Geometry: final body of the model. Coordinates: model frame, mm. A direction names the side the tool comes from. Coordinates: 2 decimals unless noted, no trailing zeros. Order: outer loops, then holes, each group sorted by start corner. A loop starts at its lowest first (then second) coordinate and runs counter-clockwise, first axis right, second up. Notation, with made-up numbers: M -25.5,57 L 2.5,57 A10 cw 2.5,76 Z; hole C -13.75,-12.5 d8. An arc over 180 degrees is marked long. Use CSV: the item, a comma, the result in double quotes. Start each with the question number.
1. Pull-direction query (Y, two-part tool) for faces 3 (the flat face through (0, 64, -6)), 4 (the flat face through (4.2, 0, 0.2)), 5 (the cylindrical face through (8.99, 7.24, 0.49)); classes: pulls with the +Y half, pulls with the -Y half, needs draft (parallel to the pull), parting line crosses it, or undercut.
2. Set-up query: faces 1 (the flat face through (1, 64, -7)), 2 (the flat face through (7, 64, 1)). Return all of +Z, -Z, +X, -X, +Y, -Y with unobstructed straight access to the full face (end or side cutting, diameter ignored); none if empty.
3. Material intervals for line 1 (Y direction, x = 8, z = 0.85); line 2 (Z direction, x = 3.5, y = 77.5), sorted ascending.
4. First-contact query: P1, Ø7, axis at y = 94.5, z = -4.5, coming from the +X side; P2, Ø4, axis at x = 5.5, y = 92.5, coming from the -Z side. Flat tips, straight axial feed; report the tip coordinate or a pass-through.
5. Section query B-B on y = 8. Return the cut outline in (x, z), and give its area (3 significant figures).
6. Section query A-A on x = 8. Return the cut outline in (y, z).
7. Section query D-D on z = -12.5. Return the cut outline in (x, y).
8. Section query C-C on y = 58.5. Return the cut outline in (x, z), and give its area (3 significant figures).
from build123d import *

# Parameters (mm, degrees)
SKETCH_1_W      = 15
SKETCH_1_H      = 1
EXTRUDE_1_DEPTH = 130
SKETCH_3_W      = 1
SKETCH_3_H      = 130
EXTRUDE_2_DEPTH = 14
M3X0_5_2_D      = 2.5


with BuildPart() as part:
    # ｽｹｯﾁ1 → ﾎﾞｽ - 押し出し1 (new body)
    with BuildSketch(Plane(origin=(0, 0, 0), x_dir=(1, 0, 0), z_dir=(0, 1, 0))):
        with Locations((7.5, -0.5)):
            Rectangle(SKETCH_1_W, SKETCH_1_H)
    extrude(amount=EXTRUDE_1_DEPTH)

    # ｽｹｯﾁ3 → ﾎﾞｽ - 押し出し2 (add)
    with BuildSketch(Plane(origin=(0, 0, 0), x_dir=(-1, 0, 0), z_dir=(0, 0, -1))):
        with Locations((-0.5, 65)):
            Rectangle(SKETCH_3_W, SKETCH_3_H)
    extrude(amount=EXTRUDE_2_DEPTH)

    # M3x0.5 ねじ穴2 (through all)
    with Locations(Plane.XY.offset(1)):
        with Locations((8, 8)):
            Hole(M3X0_5_2_D / 2)


solid = part.part
Results list:
1,face 3,"needs draft"
1,face 4,"pulls with the -Y half"
1,face 5,"undercut"
2,face 1,"-Z, +X, +Y, -Y"
2,face 2,"+Z, +X, -X, +Y, -Y"
3,line 1,"y = 0 to 6.75, 9.25 to 130"
3,line 2,"z = 0 to 1"
4,P1,"stops at x = 1"
4,P2,"stops at z = 0"
5,outline,"M 0,-14 L 1,-14 L 1,0 L 6.75,0 L 6.75,1 L 0,1 Z; M 9.25,0 L 15,0 L 15,1 L 9.25,1 Z"
5,area,"26.5 mm²"
6,outline,"M 0,0 L 6.75,0 L 6.75,1 L 0,1 Z; M 9.25,0 L 130,0 L 130,1 L 9.25,1 Z"
7,outline,"M 0,0 L 1,0 L 1,130 L 0,130 Z"
8,outline,"M 0,-14 L 1,-14 L 1,0 L 15,0 L 15,1 L 0,1 Z"
8,area,"29.0 mm²"
